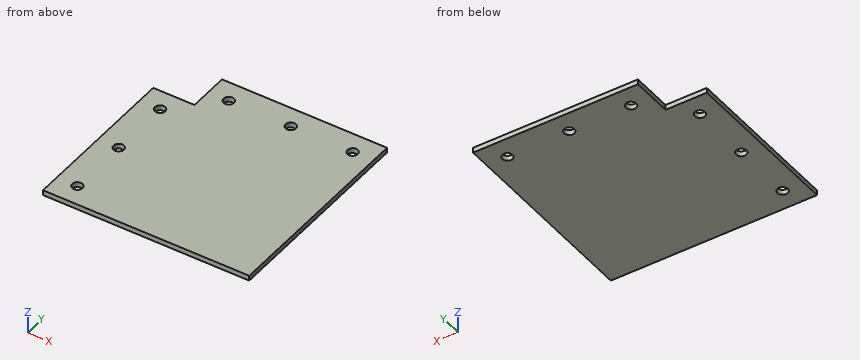
from build123d import *

# Parameters (mm, degrees)
SKETCH1_R           = 3.175
BOSS_EXTRUDE1_DEPTH = 3.175


with BuildPart() as part:
    # Sketch1 → Boss-Extrude1 (new body)
    with BuildSketch(Plane.XY):
        Polygon((0, 0), (127, 0), (127, 127), (25.4, 127), (25.4, 101.6), (0, 101.6), align=None)
        with Locations((12.7, 88.9)):
            Circle(SKETCH1_R, mode=Mode.SUBTRACT)
        with Locations((12.7, 50.8)):
            Circle(SKETCH1_R, mode=Mode.SUBTRACT)
        with Locations((12.7, 12.7)):
            Circle(SKETCH1_R, mode=Mode.SUBTRACT)
        with Locations((38.1, 114.3)):
            Circle(SKETCH1_R, mode=Mode.SUBTRACT)
        with Locations((76.2, 114.3)):
            Circle(SKETCH1_R, mode=Mode.SUBTRACT)
        with Locations((114.3, 114.3)):
            Circle(SKETCH1_R, mode=Mode.SUBTRACT)
    extrude(amount=BOSS_EXTRUDE1_DEPTH)


solid = part.part
Source: CAD feature listing. Evaluate the final solid. Frame: model axes, mm. Give positions to 0.01 mm unless a question says otherwise; leave off trailing zeros. Order: outer loops, then holes, each group sorted by start corner. A loop starts at its lowest first (then second) coordinate and runs counter-clockwise, first axis right, second up. Notation, with made-up numbers: (-32.75, 2) -> (7.25, 2) arc R14 ccw to (7.25, 26) -> close; hole circle Ø11 at (-6.75, 47.5). An arc over 180 degrees is marked (long way). Write item = value, one per line.
Item 1: Section query A-A (x = 12.7). Output: boundary loops of the cut face in (y, z) (3 decimals), then the cut area to 3 significant figures.
Check result:
outline = (0, 0) -> (9.525, 0) -> (9.525, 3.175) -> (0, 3.175) -> close; (15.875, 0) -> (47.625, 0) -> (47.625, 3.175) -> (15.875, 3.175) -> close; (53.975, 0) -> (85.725, 0) -> (85.725, 3.175) -> (53.975, 3.175) -> close; (92.075, 0) -> (101.6, 0) -> (101.6, 3.175) -> (92.075, 3.175) -> close
area = 262 mm²
Item 2: Contact query for flat-ended pins moving along their axis: pin 1 (1 mm diameter, centred on y = 116, z = 1.5, fed in from -X); pin 2 (1.6 mm diameter, centred on x = 16, z = 2, fed in from +Y). Output: stop coordinate, or through.
Check result:
pin_1 = 25.4
pin_2 = 101.6
Item 3: Ray query, probe 1 along Y at (x, z) = (12.7, 2) (3 decimals); probe 2 along X at (y, z) = (118, 2.35); probe 3 along Y at (x, z) = (78, 2.15). Return the intervals inside material, ascending.
Check result:
probe_1 = 0 to 9.525, 15.875 to 47.625, 53.975 to 85.725, 92.075 to 101.6
probe_2 = 25.4 to 127
probe_3 = 0 to 111.68, 116.92 to 127
Item 4: Section query C-C (y = 114.3). Output: boundary loops of the cut face in (x, z) (3 decimals), then the cut area to 3 significant figures.
Check result:
outline = (25.4, 0) -> (34.925, 0) -> (34.925, 3.175) -> (25.4, 3.175) -> close; (41.275, 0) -> (73.025, 0) -> (73.025, 3.175) -> (41.275, 3.175) -> close; (79.375, 0) -> (111.125, 0) -> (111.125, 3.175) -> (79.375, 3.175) -> close; (117.475, 0) -> (127, 0) -> (127, 3.175) -> (117.475, 3.175) -> close
area = 262 mm²
Item 5: Section query B-B (y = 50.8). Output: boundary loops of the cut face in (x, z) (3 decimals).
Check result:
outline = (0, 0) -> (9.525, 0) -> (9.525, 3.175) -> (0, 3.175) -> close; (15.875, 0) -> (127, 0) -> (127, 3.175) -> (15.875, 3.175) -> close
Item 6: Section query D-D (x = 76.2). Output: boundary loops of the cut face in (y, z) (3 decimals).
Check result:
outline = (0, 0) -> (111.125, 0) -> (111.125, 3.175) -> (0, 3.175) -> close; (117.475, 0) -> (127, 0) -> (127, 3.175) -> (117.475, 3.175) -> close
